Could you check a few things on this drawing? It's one solid part, dimensions in mm from its lowest x, y, z. A direction names the side the tool comes from. Give positions to 0.01 mm unless a question says otherwise; leave off trailing zeros. Order: outer loops, then holes, each group sorted by start corner. A loop starts at its lowest first (then second) coordinate and runs counter-clockwise, first axis right, second up. Notation, with made-up numbers: M -22.5,12 L -10.5,12 A23 cw -10.5,35 Z; hole C 84.5,-5.5 d7. An arc over 180 degrees is marked long. Use one line per item in the form item = value. Start each with the question number.
1. I want a section at D-D, the plane y = 5. List the corners of the cut face in (x, z) for me.
2. I want a section at B-B, the plane z = 5.75. List the corners of the cut face in (x, y) for me, and give its area (3 significant figures).
3. I want a section at A-A, the plane y = 1.5. List the corners of the cut face in (x, z) for me.
4. I need wall thicknesses on L1, parallel to X at y = 1, z = 6; L2, parallel to Y at x = 7.5, z = 6.25. Which ranges of each line are inside material? Lowest first, please.
5. We'd pull the mould along Z, two halves only. Please class the marked faces 3, 4, 5 and 6: +Z half, -Z half, draft (parallel to the pull), parting line (faces both ways), or undercut.
6. For the marked faces 1 and 2, which set-ups out of +Z, -Z, +X, -X, +Y, -Y let a thin tool reach every point of the face, with its end or its side?
7. I want a section at C-C, the plane x = 2.25. List the corners of the cut face in (y, z) for me.
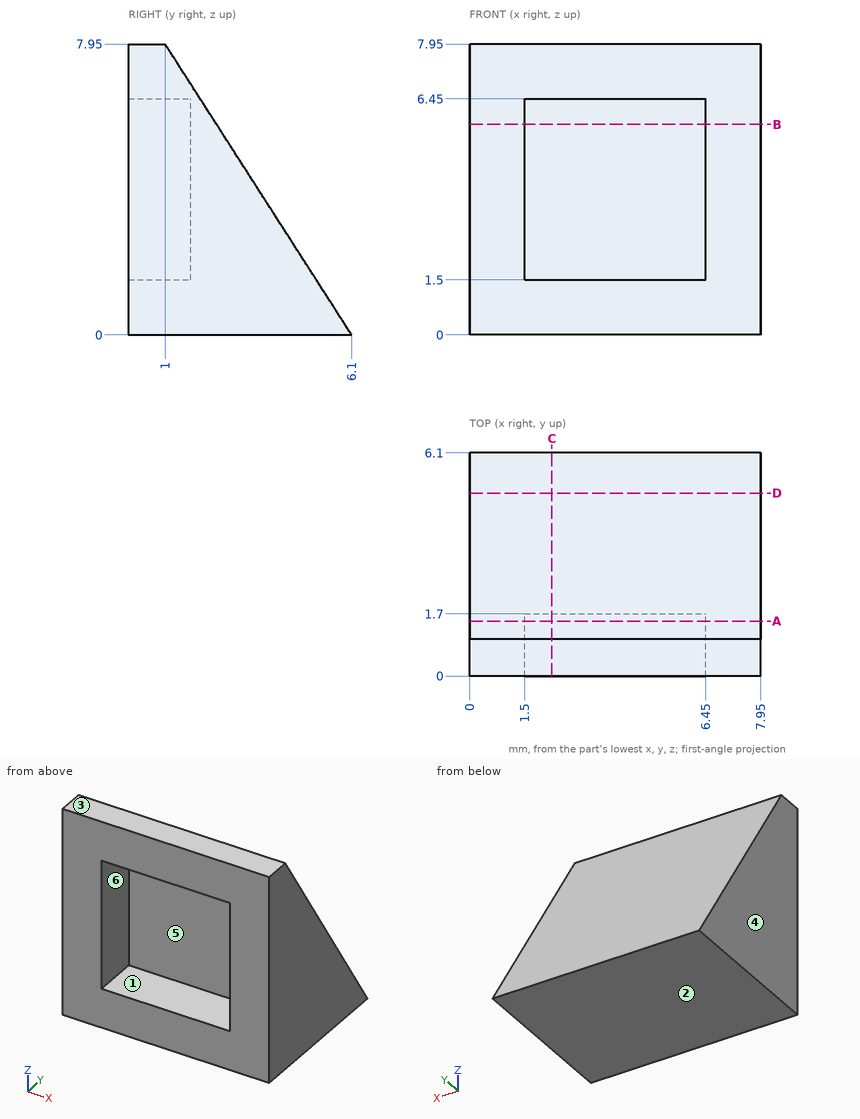
Check result:
q1.outline = M 0,0 L 7.95,0 L 7.95,1.71 L 0,1.71 Z
q2.outline = M 0,0 L 1.5,0 L 1.5,1.7 L 6.45,1.7 L 6.45,0 L 7.95,0 L 7.95,2.41 L 0,2.41 Z
q2.area = 10.8 mm2
q3.outline = M 0,0 L 7.95,0 L 7.95,7.17 L 0,7.17 Z; hole M 1.5,1.5 L 6.45,1.5 L 6.45,6.45 L 1.5,6.45 Z
q4.L1 = 0 to 1.5, 6.45 to 7.95
q4.L2 = 0 to 2.09
q5.face_3 = +Z half
q5.face_4 = draft
q5.face_5 = undercut
q5.face_6 = undercut
q6.face_1 = -Y
q6.face_2 = -Z, +X, -X, +Y, -Y
q7.outline = M 0,0 L 6.1,0 L 1,7.95 L 0,7.95 L 0,6.45 L 1.7,6.45 L 1.7,1.5 L 0,1.5 Z
